Could you check a few things on this drawing? It's one solid part, dimensions in mm from its lowest x, y, z. Give positions to 0.01 mm unless a question says otherwise; leave off trailing zeros. Order: outer loops, then holes, each group sorted by start corner. A loop starts at its lowest first (then second) coordinate and runs counter-clockwise, first axis right, second up. Notation, with made-up numbers: (60, 39.25) -> (106, 39.25) arc R17 cw to (106, 61.25) -> close; hole circle Ø2 at (62, -36). An arc over 180 degrees is marked (long way). Answer as a JSON object with one key per item and string values.
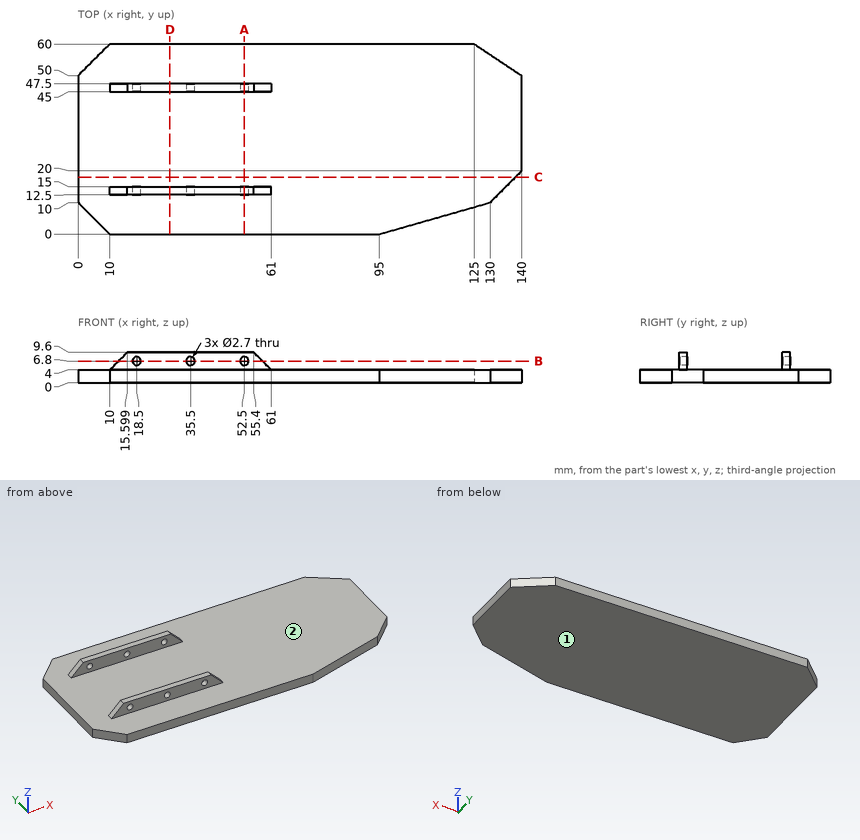
1. Will these pins go through, and if not, where does the flat tip stop? pin 1 Ø18 at (x, y) = (45, 24.5) entering from +Z; pin 2 Ø1.6 at (x, z) = (35.5, 6.8) entering from +Y; pin 3 Ø4.5 at (x, z) = (47.5, 6.5) entering from +Y; pin 4 Ø3.5 at (x, z) = (18.5, 6.8) entering from -Y.
Worked answers:
{"pin 1": "z = 4", "pin 2": "through", "pin 3": "y = 47.5", "pin 4": "y = 12.5"}
2. If we section it at D-D on x = 29: Please give me the cut outline in (y, z).
Worked answers:
{"outline": "(0, 0) -> (60, 0) -> (60, 4) -> (47.5, 4) -> (47.5, 9.6) -> (45, 9.6) -> (45, 4) -> (15, 4) -> (15, 9.6) -> (12.5, 9.6) -> (12.5, 4) -> (0, 4) -> close"}
3. If we mould it in two halves opening along Y, with no side actions, what happens to the marked faces 1 and 2? For each: +Y half, -Y half, draft (parallel to the pull), parting line (faces both ways), or undercut.
Worked answers:
{"face 1": "draft", "face 2": "undercut"}
4. If we section it at B-B on z = 6.8: Count the separate pieces of the cut face and the enclosed holes in it.
Worked answers:
{"separate pieces": "8", "enclosed holes": "0"}
5. Please list where these lines run through material, in increasing order: L1, parallel to Y at x = 49.5, z = 6; L2, parallel to Z at x = 18.5, y = 14.3; L3, parallel to Z at x = 91.5, y = 54.
Worked answers:
{"L1": "12.5 to 15, 45 to 47.5", "L2": "0 to 5.45, 8.15 to 9.6", "L3": "0 to 4"}
6. If we section it at A-A on x = 52.5: Please give me the cut outline in (y, z).
Worked answers:
{"outline": "(0, 0) -> (60, 0) -> (60, 4) -> (47.5, 4) -> (47.5, 5.45) -> (45, 5.45) -> (45, 4) -> (15, 4) -> (15, 5.45) -> (12.5, 5.45) -> (12.5, 4) -> (0, 4) -> close; (12.5, 8.15) -> (15, 8.15) -> (15, 9.6) -> (12.5, 9.6) -> close; (45, 8.15) -> (47.5, 8.15) -> (47.5, 9.6) -> (45, 9.6) -> close"}
7. If we section it at C-C on y = 18: Please give me the cut outline in (x, z), then the cut area to 3 significant figures.
Worked answers:
{"outline": "(0, 0) -> (138, 0) -> (138, 4) -> (0, 4) -> close", "area": "552 mm²"}
